Check sheet for the modelled part. Datum: model origin and axes. Units: mm. Round coordinates to 2 decimals unless told otherwise and drop trailing zeros. Write each loop counter-clockwise with the first axis right and the second up, starting at its lowest first coordinate (ties: lowest second). Pieces come first, ordered by that corner, then holes. Notation, with made-up numbers: (10.25, 69.25) - (61.25, 69.25) arc R17 cw to (61.25, 75.25) - close; hole circle Ø6 at (7.5, 13). An arc over 180 degrees is marked (long way). Use one line per item in the form item = value. Start each with the question number.
1) Section check B-B (y = 0.25). Record the boundary of the cut face in (x, z), then the cut area to 3 significant figures.
2) Section check D-D (z = 14). Record the boundary of the cut face in (x, y), then the cut area to 3 significant figures.
3) Gauge pin test, flat end, axial feed: P1, Ø5.5, axis at x = 0, y = 0, coming from the -Z side. Record the tip position at first contact, or that the pin passes through.
4) Scan lines: probe 1 along Z at (x, y) = (0, 4.5); probe 2 along X at (y, z) = (0, 25); probe 3 along X at (y, z) = (0.5, 3.6). Record each from-to range of solid material in increasing order.
5) Section check C-C (x = 0). Record the boundary of the cut face in (y, z), then the cut area to 3 significant figures.
6) Section check A-A (z = 3.6). Record the boundary of the cut face in (x, y), then the cut area to 3 significant figures.
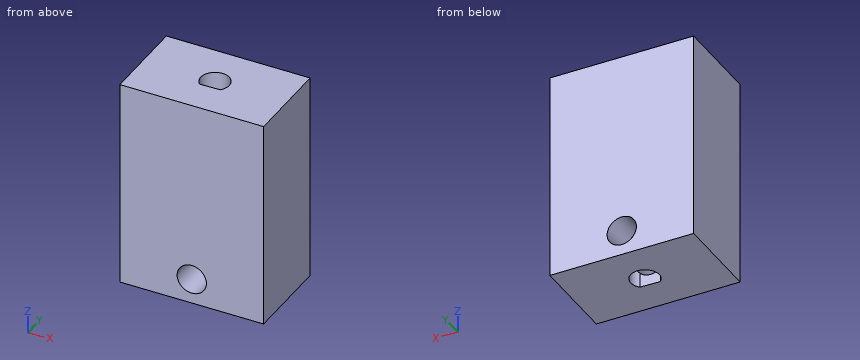
from build123d import *

# Parameters (mm, degrees)
SKETCH_2_W          = 20.6
SKETCH_2_H          = 12.6
EXTRUDE_1_DEPTH     = 30
CUT_EXTRUDE_1_DEPTH = 30
SKETCH_4_R          = 2.1
CUT_EXTRUDE_3_DEPTH = 6
SKETCH_6_R          = 2.1
CUT_EXTRUDE_4_DEPTH = 30


with BuildPart() as part:
    # Эскиз2 → Бобышка-Вытянуть1 (new body)
    with BuildSketch(Plane.XY):
        Rectangle(SKETCH_2_W, SKETCH_2_H)
    extrude(amount=EXTRUDE_1_DEPTH)

    # Эскиз3 → Вырез-Вытянуть1 (cut)
    with BuildSketch(Plane.XY.offset(30)):
        with BuildLine():
            Line((-1.408154236, -1.489832758), (1.488994806, -1.409040265))
            ThreePointArc((1.488994806, -1.409040265), (-0.05714592, 2.049203344), (-1.408154236, -1.489832758))
        make_face()
    extrude(amount=-CUT_EXTRUDE_1_DEPTH, mode=Mode.SUBTRACT)

    # Эскиз4 → Вырез-Вытянуть3 (cut)
    with BuildSketch(Plane.XZ.offset(6.3)):
        with Locations(Location((0, 3.6, 0), (0, 0, 270))):
            Circle(SKETCH_4_R)
    extrude(amount=-CUT_EXTRUDE_3_DEPTH, mode=Mode.SUBTRACT)

    # Эскиз6 → Вырез-Вытянуть4 (cut)
    with BuildSketch(Plane.XZ.offset(6.3)):
        with Locations(Location((0, 3.6, 0), (0, 0, 270))):
            Circle(SKETCH_6_R)
    extrude(amount=-CUT_EXTRUDE_4_DEPTH, mode=Mode.SUBTRACT)


solid = part.part
Results are:
q1.outline = (-10.3, 0) - (-2.03, 0) - (-2.03, 3.08) arc R2.1 cw to (-2.03, 4.12) - (-2.03, 30) - (-10.3, 30) - close; (2.03, 0) - (10.3, 0) - (10.3, 30) - (2.03, 30) - (2.03, 4.12) arc R2.1 cw to (2.03, 3.08) - close
q1.area = 496 mm²
q2.outline = (-10.3, -6.3) - (10.3, -6.3) - (10.3, 6.3) - (-10.3, 6.3) - close; hole (-1.41, -1.49) - (1.49, -1.41) arc R2.05 ccw (long way) to start
q2.area = 248 mm²
q3.P1 = 0
q4.probe_1 = 0 to 1.5, 5.7 to 30
q4.probe_2 = -10.3 to -2.05, 2.05 to 10.3
q4.probe_3 = -10.3 to -2.1, 2.1 to 10.3
q5.outline = (-6.3, 0) - (-1.45, 0) - (-1.45, 1.5) - (-6.3, 1.5) - close; (-6.3, 5.7) - (-1.45, 5.7) - (-1.45, 30) - (-6.3, 30) - close; (2.05, 0) - (6.3, 0) - (6.3, 1.5) - (2.05, 1.5) - close; (2.05, 5.7) - (6.3, 5.7) - (6.3, 30) - (2.05, 30) - close
q5.area = 235 mm²
q6.outline = (-10.3, -6.3) - (-2.1, -6.3) - (-2.1, 6.3) - (-10.3, 6.3) - close; (2.1, -6.3) - (10.3, -6.3) - (10.3, 6.3) - (2.1, 6.3) - close
q6.area = 207 mm²
